from build123d import *

# Parameters (mm, degrees)
SKETCH1_W           = 200
SKETCH1_H           = 46
BOSS_EXTRUDE1_DEPTH = 6
SKETCH2_W           = 40
SKETCH2_H           = 6
CUT_EXTRUDE1_DEPTH  = 6
SKETCH3_W           = 10
SKETCH3_H           = 6
CUT_EXTRUDE2_DEPTH  = 10
SKETCH4_W           = 30
SKETCH4_H           = 6
CUT_EXTRUDE3_DEPTH  = 10


with BuildPart() as part:
    # Sketch1 → Boss-Extrude1 (new body)
    with BuildSketch(Plane.XY):
        Rectangle(SKETCH1_W, SKETCH1_H)
    extrude(amount=BOSS_EXTRUDE1_DEPTH)

    # Sketch2 → Cut-Extrude1 (cut)
    with BuildSketch(Plane.XY.offset(6)):
        with Locations((0, -20)):
            Rectangle(SKETCH2_W, SKETCH2_H)
        with Locations((-80, -20)):
            Rectangle(SKETCH2_W, SKETCH2_H)
        with Locations((80, -20)):
            Rectangle(SKETCH2_W, SKETCH2_H)
    extrude(amount=-CUT_EXTRUDE1_DEPTH, mode=Mode.SUBTRACT)

    # Sketch3 → Cut-Extrude2 (cut)
    with BuildSketch(Plane.XY.offset(6)):
        with Locations((-95, -8)):
            Rectangle(SKETCH3_W, SKETCH3_H)
        with Locations((-75, -8)):
            Rectangle(SKETCH3_W, SKETCH3_H)
    extrude(amount=-CUT_EXTRUDE2_DEPTH, mode=Mode.SUBTRACT)

    # Sketch4 → Cut-Extrude3 (cut)
    with BuildSketch(Plane.XY.offset(6)):
        with Locations((-85, 4)):
            Rectangle(SKETCH4_W, SKETCH4_H)
    extrude(amount=-CUT_EXTRUDE3_DEPTH, mode=Mode.SUBTRACT)


solid = part.part
The model under review builds one solid part; all positions refer to its coordinate system, in mm. A direction names the side the tool comes from. Round coordinates to 2 decimals unless told otherwise and drop trailing zeros. Loops run counter-clockwise (first coordinate to the right, second up) from the corner with the lowest first, then second, coordinate; pieces in that order, holes last. Notation, with made-up numbers: (84, 60) -> (97, 60) arc R8 ccw to (97, 71) -> close; hole circle Ø6 at (84.25, 42). An arc over 180 degrees is marked (long way). Answer as CSV lines item,"result".
1) To check wall thickness, follow line 1 along Y through (x, z) = (-90.5, 2.05); line 2 along Y through (x, z) = (-87, 3.7); line 3 along X through (y, z) = (-19, 5.3). State the ranges of each line that lie inside material, in increasing order. Write a range as from..to.
Geometry results:
line 1,"y = -17..-11, -5..1, 7..23"
line 2,"y = -17..1, 7..23"
line 3,"x = -60..-20, 20..60"
2) Add section A-A on z = 3.25. Write out the cut boundary in (x, y), plus the area to 3 significant figures.
Geometry results:
outline,"(-100, -17) -> (-60, -17) -> (-60, -23) -> (-20, -23) -> (-20, -17) -> (20, -17) -> (20, -23) -> (60, -23) -> (60, -17) -> (100, -17) -> (100, 23) -> (-100, 23) -> (-100, 7) -> (-70, 7) -> (-70, 1) -> (-100, 1) -> (-100, -5) -> (-90, -5) -> (-90, -11) -> (-100, -11) -> close; hole (-80, -11) -> (-70, -11) -> (-70, -5) -> (-80, -5) -> close"
area,"8,180 mm²"
3) Draft analysis for pull direction Y (two halves, no side actions). For faces 1 (the face through (-80, -17, 3)), 2 (the face through (20, -20, 3)), 3 (the face through (-75, -5, 3)), state which applies: pulls with the +Y half, pulls with the -Y half, needs draft (parallel to the pull), parting line crosses it, or undercut.
Geometry results:
face 1,"pulls with the -Y half"
face 2,"needs draft"
face 3,"undercut"
4) Add section B-B on x = 72. Write out the cut boundary in (y, z).
Geometry results:
outline,"(-17, 0) -> (23, 0) -> (23, 6) -> (-17, 6) -> close"
5) Tool access review of faces 4 (the face through (80, -17, 3)), 5 (the face through (-85, 1, 3)), 6 (the face through (0, -17, 3)): name each direction out of +Z, -Z, +X, -X, +Y, -Y from which nothing blocks a thin tool from reaching the whole face with its end or side.
Geometry results:
face 4,"+Z, -Z, +X, -Y"
face 5,"+Z, -Z, -X"
face 6,"+Z, -Z, -Y"
6) For P1, Ø3, axis at y = 4, z = 3, coming from the -X side; P2, Ø1.8, axis at y = -20.5, z = 2, coming from the -X side; P3, Ø1.8, axis at x = -81.5, z = 2.5, coming from the -Y side, all flat-tipped, find the tip position at first contact; note any pin that passes through.
Geometry results:
P1,"stops at x = -70"
P2,"stops at x = -60"
P3,"stops at y = -17"
